Build history of the part. All positions in model axes, mm. Face numbers are marked on the shaded views. A direction names the side the tool comes from. Round coordinates to 2 decimals unless told otherwise and drop trailing zeros. Loops run counter-clockwise (first coordinate to the right, second up) from the corner with the lowest first, then second, coordinate; pieces in that order, holes last. Notation, with made-up numbers: (84, 6.5) - (142, 6.5) arc R19 cw to (142, 31.5) - close; hole circle Ø7 at (66, 63). An arc over 180 degrees is marked (long way). Answer as CSV lines item,"result". Start each with the question number.
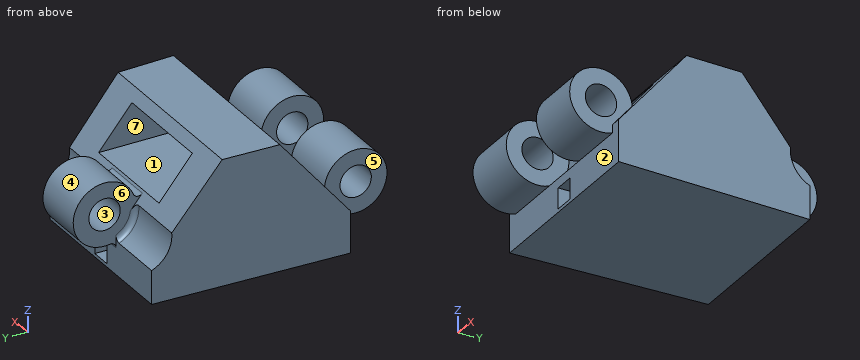
```python
from build123d import *

# Parameters (mm, degrees)
BOSS_EXTRUDE2_DEPTH             = 12
CUT_EXTRUDE2_DEPTH              = 22.571014648
CUT_EXTRUDE2_DEPTH_BACK         = 22.571014648
BOSS_EXTRUDE3_DEPTH             = 2.5
CUT_EXTRUDE3_DEPTH              = 25.679395228
CUT_EXTRUDE3_DEPTH_BACK         = 25.679395228
SKETCH19_R                      = 3
SKETCH19_R_2                    = 1.5
BOSS_EXTRUDE4_DEPTH             = 8
SKETCH19_3_R                    = 3
CUT_EXTRUDE4_DEPTH              = 2.5
CUT_EXTRUDE5_START              = 10
SKETCH20_R                      = 3
CUT_EXTRUDE5_DEPTH              = 10
SKETCH21_R                      = 3
CUT_EXTRUDE6_DEPTH              = 10
FILLET6_R                       = 0.5
FILLET7_R                       = 0.5
FILLET8_R                       = 0.5
CUT_EXTRUDE8_DEPTH              = 25.679395276
CUT_EXTRUDE8_DEPTH_BACK         = 25.679395276
CUT_EXTRUDE9_DEPTH              = 24.907546424
CUT_EXTRUDE9_DEPTH_BACK         = 24.907546424
SKETCH26_R                      = 3
SKETCH27_R                      = 3
SKETCH27_R_2                    = 1.5
BOSS_EXTRUDE6_DEPTH             = 2.5
FILLET9_R                       = 0.5
FILLET10_R                      = 0.5
CUT_EXTRUDE10_REACH             = 22.744
SKETCH29_W                      = 10
SKETCH29_H                      = 3.849855631
CUT_EXTRUDE10_DIRECTION_2_REACH = 22.744
SKETCH30_W                      = 2
SKETCH30_H                      = 21.746191479
CUT_EXTRUDE11_DEPTH             = 1


with BuildPart() as part:
    # Sketch1 → Boss-Extrude2 (new body)
    with BuildSketch(Plane.XY):
        Polygon((-8, -14.5), (-6.966131725, 15.482179981), (9.033868275, 15.482179981), (10.06773655, -14.5), align=None)
    extrude(amount=BOSS_EXTRUDE2_DEPTH)

    # Sketch16 → Cut-Extrude2 (cut, two sides: drawn at the far end of the back side and taken through both)
    with BuildSketch(Plane(origin=(1.033868275, 0, 0), x_dir=(0, 0, -1), z_dir=(1, 0, 0)).offset(-CUT_EXTRUDE2_DEPTH_BACK)):
        Polygon((-12, 15.482179981), (-4, 15.482179981), (-12, 8.852541981), align=None)
    extrude(amount=CUT_EXTRUDE2_DEPTH + CUT_EXTRUDE2_DEPTH_BACK, mode=Mode.SUBTRACT)

    # Sketch17 → Boss-Extrude3 (add, symmetric)
    with BuildSketch(Plane(origin=(1.033868275, 0, 0), x_dir=(0, 0, -1), z_dir=(1, 0, 0))):
        with BuildLine():
            ThreePointArc((-8.791057147, 15.482179981), (-6, 13.582179981), (-3.208942853, 15.482179981))
            Line((-3.208942853, 15.482179981), (-4.980196097, 15.482179981))
            ThreePointArc((-4.980196097, 15.482179981), (-6, 15.082179981), (-7.019803903, 15.482179981))
            Line((-7.019803903, 15.482179981), (-8.791057147, 15.482179981))
        make_face()
        with BuildLine():
            Line((-4.980196097, 15.482179981), (-3.208942853, 15.482179981))
            ThreePointArc((-3.208942853, 15.482179981), (-3.05269857, 16.022345828), (-3, 16.582179981))
            ThreePointArc((-3, 16.582179981), (-6.559834153, 19.529481411), (-8.791057147, 15.482179981))
            Line((-8.791057147, 15.482179981), (-7.019803903, 15.482179981))
            ThreePointArc((-7.019803903, 15.482179981), (-6.600122548, 17.956899198), (-4.5, 16.582179981))
            ThreePointArc((-4.5, 16.582179981), (-4.625280782, 15.982057432), (-4.980196097, 15.482179981))
        make_face()
    extrude(amount=BOSS_EXTRUDE3_DEPTH, both=True)

    # Sketch18 → Cut-Extrude3 (cut, two sides: drawn at the far end of the back side and taken through both)
    with BuildSketch(Plane(origin=(1.033868275, 0, 0), x_dir=(0, 0, -1), z_dir=(1, 0, 0)).offset(-CUT_EXTRUDE3_DEPTH_BACK)):
        Polygon((-12, -7.870362001), (-12, -14.5), (-4, -14.5), align=None)
    extrude(amount=CUT_EXTRUDE3_DEPTH + CUT_EXTRUDE3_DEPTH_BACK, mode=Mode.SUBTRACT)

    # Sketch19 → Boss-Extrude4 (add, symmetric)
    with BuildSketch(Plane(origin=(1.033868275, 0, 0), x_dir=(0, 0, -1), z_dir=(1, 0, 0))):
        with Locations((-6, -15.6)):
            Circle(SKETCH19_R)
        with Locations((-6, -15.6)):
            Circle(SKETCH19_R_2, mode=Mode.SUBTRACT)
    extrude(amount=BOSS_EXTRUDE4_DEPTH, both=True)

    # Sketch19_3 → Cut-Extrude4 (cut, symmetric)
    with BuildSketch(Plane(origin=(1.033868275, 0, 0), x_dir=(0, 0, -1), z_dir=(1, 0, 0))):
        with Locations((-6, -15.6)):
            Circle(SKETCH19_3_R)
    extrude(amount=CUT_EXTRUDE4_DEPTH, both=True, mode=Mode.SUBTRACT)

    # Sketch20 → Cut-Extrude5 (cut)
    with BuildSketch(Plane(origin=(3.533868275, 0, 0), x_dir=(0, 0, -1), z_dir=(1, 0, 0)).offset(CUT_EXTRUDE5_START)):
        with Locations((-6, 16.582179981)):
            Circle(SKETCH20_R)
    extrude(amount=-CUT_EXTRUDE5_DEPTH, mode=Mode.SUBTRACT)

    # Sketch21 → Cut-Extrude6 (cut)
    with BuildSketch(Plane.ZY.offset(1.466131725)):
        with Locations((6, 16.582179981)):
            Circle(SKETCH21_R)
    extrude(amount=CUT_EXTRUDE6_DEPTH, mode=Mode.SUBTRACT)

    # Fillet6
    fillet6_edges = [part.edges().sort_by_distance(p)[0] for p in [
        (1.033868275, 13.595018046, 6.277242812),
    ]]
    fillet(fillet6_edges, radius=FILLET6_R)

    # Fillet7
    fillet7_edges = [part.edges().sort_by_distance(p)[0] for p in [
        (1.033868275, 15.482179981, 3.208942853),
    ]]
    fillet(fillet7_edges, radius=FILLET7_R)

    # Fillet8
    fillet8_edges = [part.edges().sort_by_distance(p)[0] for p in [
        (3.533868275, 14.026824951, 4.42832552),
        (-1.466131725, 14.026824951, 4.42832552),
    ]]
    fillet(fillet8_edges, radius=FILLET8_R)

    # Sketch23 → Cut-Extrude8 (cut, two sides: drawn at the far end of the back side and taken through both)
    with BuildSketch(Plane(origin=(1.033868275, 0, 0), x_dir=(0, 0, -1), z_dir=(1, 0, 0)).offset(-CUT_EXTRUDE8_DEPTH_BACK)):
        Polygon((0, 4.167360981), (0, 23.255957395), (-12, 23.255957395), (-12, -2.462277018), (-4, 4.167360981), align=None)
    extrude(amount=CUT_EXTRUDE8_DEPTH + CUT_EXTRUDE8_DEPTH_BACK, mode=Mode.SUBTRACT)

    # Sketch26 → Cut-Extrude9 (cut, two sides: drawn at the far end of the back side and taken through both)
    with BuildSketch(Plane(origin=(1.033868275, 0, 0), x_dir=(0, 0, -1), z_dir=(1, 0, 0)).offset(-CUT_EXTRUDE9_DEPTH_BACK)):
        with Locations((-6, 5.267360981)):
            Circle(SKETCH26_R)
    extrude(amount=CUT_EXTRUDE9_DEPTH + CUT_EXTRUDE9_DEPTH_BACK, mode=Mode.SUBTRACT)

    # Sketch27 → Boss-Extrude6 (add, symmetric)
    with BuildSketch(Plane(origin=(1.033868275, 0, 0), x_dir=(0, 0, -1), z_dir=(1, 0, 0))):
        with Locations((-6, 5.267360981)):
            Circle(SKETCH27_R)
        with Locations((-6, 5.267360981)):
            Circle(SKETCH27_R_2, mode=Mode.SUBTRACT)
    extrude(amount=BOSS_EXTRUDE6_DEPTH, both=True)

    # Fillet9
    fillet9_edges = [part.edges().sort_by_distance(p)[0] for p in [
        (1.033868275, 4.167360981, 3.208942853),
        (1.033868275, 2.280199046, 6.277242812),
    ]]
    fillet(fillet9_edges, radius=FILLET9_R)

    # Fillet10
    fillet10_edges = [part.edges().sort_by_distance(p)[0] for p in [
        (3.533868275, 2.712005951, 4.42832552),
        (-1.466131725, 2.712005951, 4.42832552),
    ]]
    fillet(fillet10_edges, radius=FILLET10_R)

    # Cut-Extrude10: up to this plane
    cut_extrude10_end = Plane(origin=(-8, -10.561614049, 8.752459729), z_dir=(0, 0.769971126082772, -0.6380787294674758))
    # Sketch29 → Cut-Extrude10 (cut, up to the surface)
    with BuildSketch(Plane(origin=(0, -5, 0), x_dir=(1, 0, 0), z_dir=(0, 1, 0)), mode=Mode.PRIVATE) as cut_extrude10_sk1:
        with Locations((1.033868275, -9.151106834)):
            Rectangle(SKETCH29_W, SKETCH29_H)
    cut_extrude10_tool1 = split(extrude(cut_extrude10_sk1.sketch, amount=-CUT_EXTRUDE10_REACH, mode=Mode.PRIVATE), bisect_by=cut_extrude10_end, keep=Keep.BOTH, mode=Mode.PRIVATE)
    add(cut_extrude10_tool1.solids().sort_by_distance((1.033868, -5, 9.151107))[0], mode=Mode.SUBTRACT)

    # Cut-Extrude10 direction 2: up to this plane
    cut_extrude10_direction_2_end = Plane(origin=(-8, -2.462277018, 12), z_dir=(0, -0.769971126082772, -0.6380787294674759))
    # Sketch29 → Cut-Extrude10 direction 2 (cut, up to the surface)
    with BuildSketch(Plane(origin=(0, -5, 0), x_dir=(1, 0, 0), z_dir=(0, 1, 0)), mode=Mode.PRIVATE) as cut_extrude10_direction_2_sk1:
        with Locations((1.033868275, -9.151106834)):
            Rectangle(SKETCH29_W, SKETCH29_H)
    cut_extrude10_direction_2_tool1 = split(extrude(cut_extrude10_direction_2_sk1.sketch, amount=CUT_EXTRUDE10_DIRECTION_2_REACH, mode=Mode.PRIVATE), bisect_by=cut_extrude10_direction_2_end, keep=Keep.BOTH, mode=Mode.PRIVATE)
    add(cut_extrude10_direction_2_tool1.solids().sort_by_distance((1.033868, -5, 9.151107))[0], mode=Mode.SUBTRACT)

    # Sketch30 → Cut-Extrude11 (cut, symmetric)
    with BuildSketch(Plane(origin=(1.033868275, 0, 0), x_dir=(0, 0, -1), z_dir=(1, 0, 0))):
        with Locations((-1.32, -6.705734759)):
            Rectangle(SKETCH30_W, SKETCH30_H)
    extrude(amount=CUT_EXTRUDE11_DEPTH, both=True, mode=Mode.SUBTRACT)


solid = part.part
```
Q1. Band-saw the part on A-A, the plane y = -15.6. List the corners of the cut face in (x, z), then the cut area to 3 significant figures.
Q2. Tool access for the marked faces 5, 6 and 7: list every direction of +Z, -Z, +X, -X, +Y, -Y with a clear straight run to the whole face (end or side of a thin tool).
Q3. Two-plate mould, pull along Z, no slides. Class the marked faces 1, 2, 3 and 4: released by +Z, released by -Z, zero draft, split by the parting line, or undercut.
Q4. Band-saw the part on D-D, the plane y = 5.75. List the corners of the cut face in (x, z), then the cut area to 3 significant figures.
Q5. Band-saw the part on B-B, the plane z = 6. Give the number of separate pieces and of enclosed holes in the cut face, then the cut area to 3 significant figures.
Q6. Band-saw the part on C-C, the plane x = 1.75. List the corners of the cut face in (y, z).
Q7. Pin check, flat tips, straight feed: pin 1 Ø3 at (y, z) = (5, 6.5) entering from +X; pin 2 Ø5 at (x, y) = (0, -8.5) entering from +Z; pin 3 Ø5 at (y, z) = (-15.5, 7) entering from -X; pin 4 Ø1 at (x, y) = (7.5, 1) entering from +Z. Stop position of each tip, or through.
Q8. Wall check: probe 1 along Z at (x, y) = (0.75, -4.75); probe 2 along Y at (x, z) = (-5.25, 6); probe 3 along Z at (x, y) = (-3, -15.6). Give the ranges that are in metal, low to high. Write a range as [from, to].
Reported:
1,outline,"(-6.97, 3) - (-1.47, 3) - (-1.47, 4.5) - (-6.97, 4.5) - close; (-6.97, 7.5) - (-1.47, 7.5) - (-1.47, 9) - (-6.97, 9) - close; (3.53, 3) - (9.03, 3) - (9.03, 4.5) - (3.53, 4.5) - close; (3.53, 7.5) - (9.03, 7.5) - (9.03, 9) - (3.53, 9) - close"
1,area,"33.0 mm2"
2,face 5,"+Z, -X, -Y"
2,face 6,"+Z, -X, +Y"
2,face 7,"+Y"
3,face 1,"undercut"
3,face 2,"zero draft"
3,face 3,"undercut"
3,face 4,"split by the parting line"
4,outline,"(-1.47, 3.04) - (3.53, 3.04) - (3.53, 4.58) - (-1.47, 4.58) - close; (-1.47, 7.42) - (3.53, 7.42) - (3.53, 8.96) - (-1.47, 8.96) - close"
4,area,"15.4 mm2"
5,separate pieces,"4"
5,enclosed holes,"0"
5,area,"308 mm2"
6,outline,"(-14.5, 0) - (4.17, 0) - (4.17, 0.32) - (-14.5, 0.32) - close; (-14.5, 2.32) - (4.17, 2.32) - (4.17, 2.55) arc R0.5 cw to (4.75, 3.04) arc R3 ccw (long way) to (2.5, 7.16) arc R0.5 cw to (1.65, 7.03) - (1.49, 7.23) - (-11.83, 7.23) - (-12.61, 6.28) arc R3 cw to (-14.5, 3.21) - close; (-8.64, 11.08) - (-1.7, 11.08) - (-2.46, 12) - (-7.87, 12) - close; hole circle Ø3 at (5.27, 6)"
7,pin 1,"stops at x = 3.53"
7,pin 2,"stops at z = 12"
7,pin 3,"stops at x = -6.97"
7,pin 4,"stops at z = 8.43"
8,probe 1,"z = [0, 0.32], [2.32, 7.23], [11.08, 12]"
8,probe 2,"y = [-18.6, -17.1], [-14.1, 2.27]"
8,probe 3,"z = [3, 4.5], [7.5, 9]"
